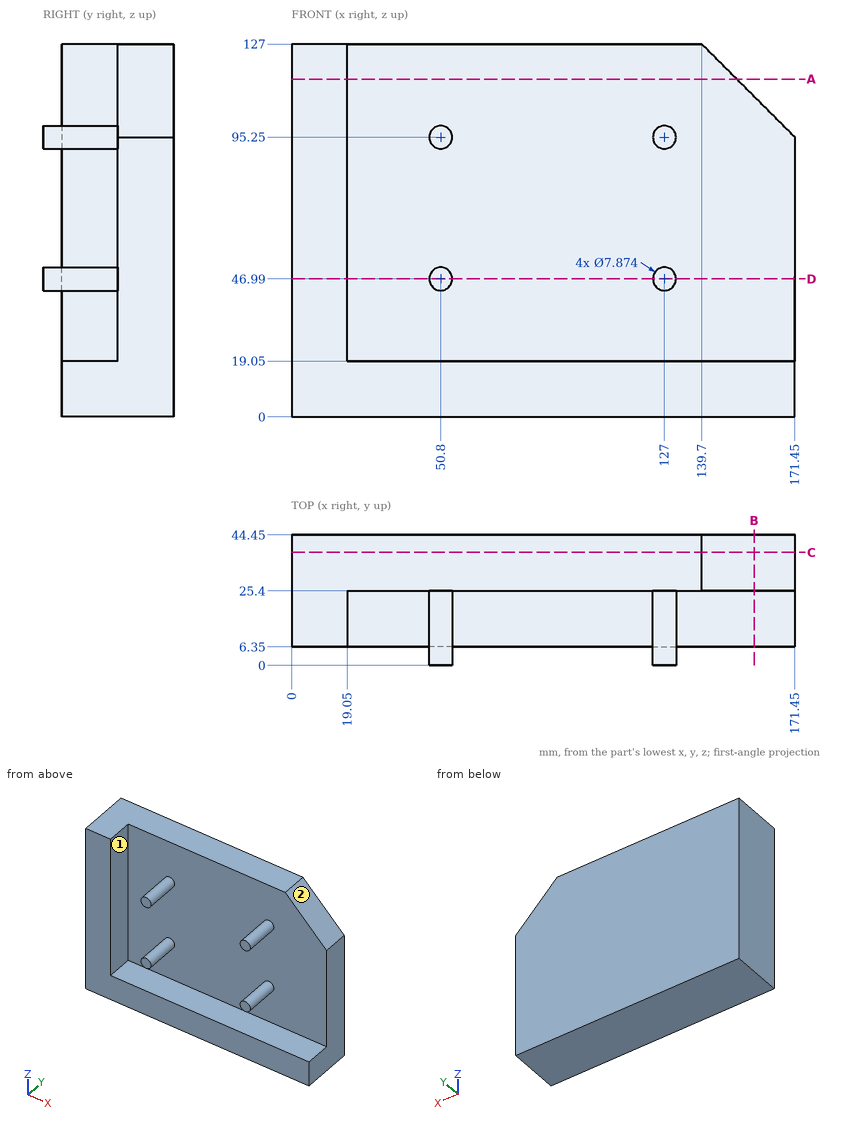
Here's the drawing with two shaded views (mm, measured from the low corner). I have some questions. A direction names the side the tool comes from. Coordinates: 2 decimals unless noted, no trailing zeros. Loops run counter-clockwise (first coordinate to the right, second up) from the corner with the lowest first, then second, coordinate; pieces in that order, holes last. Notation, with made-up numbers: (-13, -17.75) -> (27, -17.75) arc R26 cw to (27, 14.25) -> close; hole circle Ø6 at (55, -31). An arc over 180 degrees is marked (long way). Answer as a JSON object with one key per item and string values.
1) Imagine slicing it at C-C (y = 38.5). Please give me the cut outline in (x, z), then the cut area to 3 significant figures.
Results:
{"outline": "(0, 0) -> (171.45, 0) -> (171.45, 95.25) -> (139.7, 127) -> (0, 127) -> close", "area": "21,300 mm^2"}
2) For P1, Ø10, axis at y = 31.5, z = 107.5, coming from the +X side; P2, Ø5.5, axis at y = 18.5, z = 86.5, coming from the +X side; P3, Ø10, axis at x = 47, y = 5.5, coming from the +Z side, each with a flat end and sliding along its axis, tell me the tip position at first contact or that it passes through.
Results:
{"P1": "stops at x = 164.2", "P2": "stops at x = 19.05", "P3": "stops at z = 99.19"}
3) Imagine slicing it at A-A (z = 115). Please give me the cut outline in (x, y), then the cut area to 3 significant figures.
Results:
{"outline": "(0, 6.35) -> (19.05, 6.35) -> (19.05, 25.4) -> (151.7, 25.4) -> (151.7, 44.45) -> (0, 44.45) -> close", "area": "3,250 mm^2"}
4) Imagine slicing it at D-D (z = 46.99). Please give me the cut outline in (x, y).
Results:
{"outline": "(0, 6.35) -> (19.05, 6.35) -> (19.05, 25.4) -> (46.86, 25.4) -> (46.86, 0) -> (54.74, 0) -> (54.74, 25.4) -> (123.06, 25.4) -> (123.06, 0) -> (130.94, 0) -> (130.94, 25.4) -> (171.45, 25.4) -> (171.45, 44.45) -> (0, 44.45) -> close"}
5) If I drill on line 1 (Y direction, x = 127, z = 40); line 2 (X direction, y = 21, z = 36.5), over which ranges is the centre line in solid material (lowest first)?
Results:
{"line 1": "y = 25.4 to 44.45", "line 2": "x = 0 to 19.05"}
6) Imagine slicing it at B-B (x = 157.5). Please give me the cut outline in (y, z).
Results:
{"outline": "(6.35, 0) -> (44.45, 0) -> (44.45, 109.2) -> (25.4, 109.2) -> (25.4, 19.05) -> (6.35, 19.05) -> close"}
7) For the marked faces 1 and 2, which set-ups out of +Z, -Z, +X, -X, +Y, -Y let a thin tool reach every point of the face, with its end or its side?
Results:
{"face 1": "+Z, -Y", "face 2": "+Z, +X, +Y, -Y"}
